Print and shaded views of the part. All mm, measured from the part's lowest x, y and z. Coordinates: 2 decimals unless noted, no trailing zeros. Loops run counter-clockwise (first coordinate to the right, second up) from the corner with the lowest first, then second, coordinate; pieces in that order, holes last.
1) Saw through at D-D, the plane x = 120. Write the cut outline in (y, z).
2) Two-plate mould, pull along X, no slides. Class the marked faces 1, 2 and 3: +X half, -X half, draft (parallel to the pull), parting line (faces both ways), or undercut.
3) Pin check, flat tips, straight feed: pin 1 Ø6 at (x, y) = (81.5, 15) entering from -Z; pin 2 Ø6 at (x, y) = (118, 5) entering from +Z; pin 3 Ø8 at (y, z) = (2.5, 80) entering from -X. Stop position of each tip, or through.
4) Saw through at A-A, the plane x = 100. Write the cut outline in (y, z), and give its area (3 significant figures).
5) Saw through at B-B, the plane z = 50. Write the cut outline in (x, y).
6) Wall check: line 1 along Z through (x, y) = (100, 10.75); line 2 along Z through (x, y) = (80, 4); line 3 along X through (y, z) = (2, 50). Give the ranges that are in metal, low to high.
7) Saw through at C-C, the plane z = 100. Write the cut outline in (x, y).
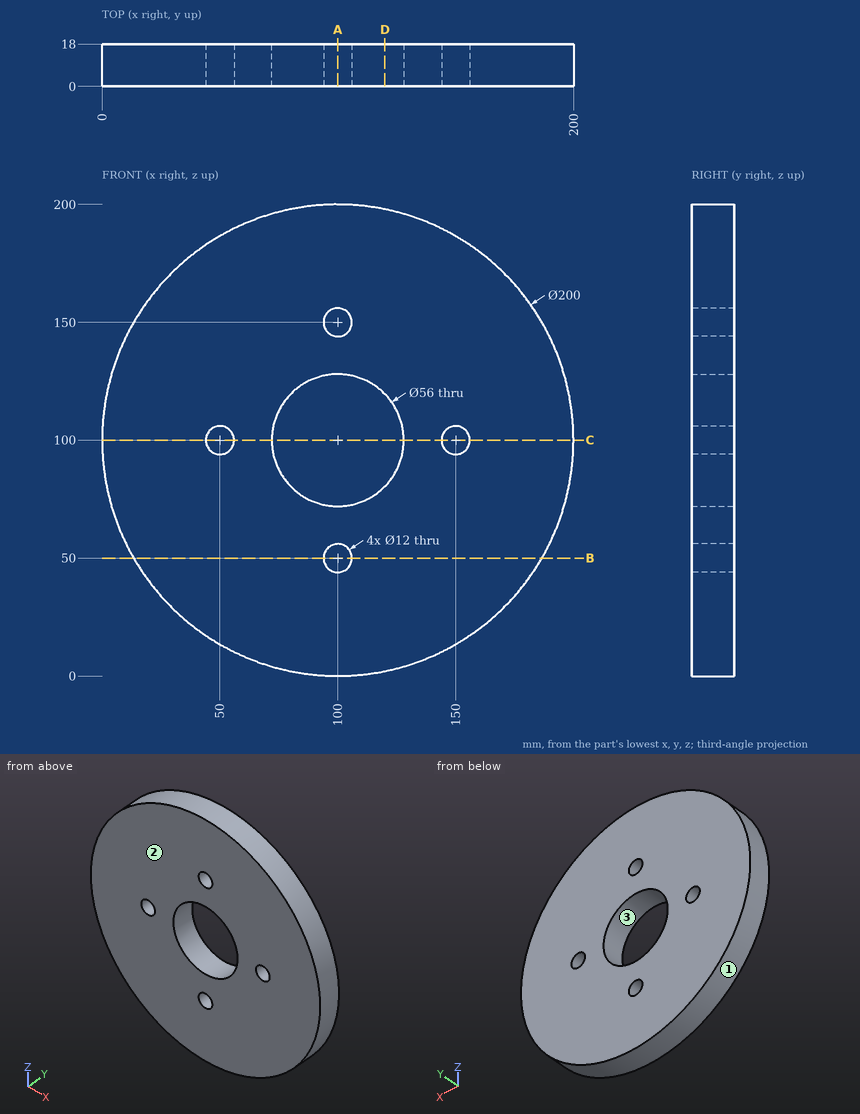
Data:
1. outline: (0, 2.02) - (18, 2.02) - (18, 80.4) - (0, 80.4) - close; (0, 119.6) - (18, 119.6) - (18, 197.98) - (0, 197.98) - close
2. face 1: parting line
2. face 2: draft
2. face 3: undercut
3. pin 1: stops at z = 1.21
3. pin 2: stops at z = 198.87
3. pin 3: stops at x = 1.29
4. outline: (0, 0) - (18, 0) - (18, 44) - (0, 44) - close; (0, 56) - (18, 56) - (18, 72) - (0, 72) - close; (0, 128) - (18, 128) - (18, 144) - (0, 144) - close; (0, 156) - (18, 156) - (18, 200) - (0, 200) - close
4. area: 2,160 mm2
5. outline: (13.4, 0) - (94, 0) - (94, 18) - (13.4, 18) - close; (106, 0) - (186.6, 0) - (186.6, 18) - (106, 18) - close
6. line 1: z = 0 to 44, 56 to 72, 128 to 144, 156 to 200
6. line 2: z = 2.02 to 80.4, 119.6 to 197.98
6. line 3: x = 13.4 to 94, 106 to 186.6
7. outline: (0, 0) - (44, 0) - (44, 18) - (0, 18) - close; (56, 0) - (72, 0) - (72, 18) - (56, 18) - close; (128, 0) - (144, 0) - (144, 18) - (128, 18) - close; (156, 0) - (200, 0) - (200, 18) - (156, 18) - close
